Part model, mm, in its own coordinate system. Give positions to 0.01 mm unless a question says otherwise; leave off trailing zeros. Loops run counter-clockwise (first coordinate to the right, second up) from the corner with the lowest first, then second, coordinate; pieces in that order, holes last. Notation, with made-up numbers: (-27.75, -26.75) -> (2.25, -26.75) arc R24 cw to (2.25, 4.25) -> close; hole circle Ø3 at (53, -16.5). An arc over 180 degrees is marked (long way). One line per question, with ' | ' between items.
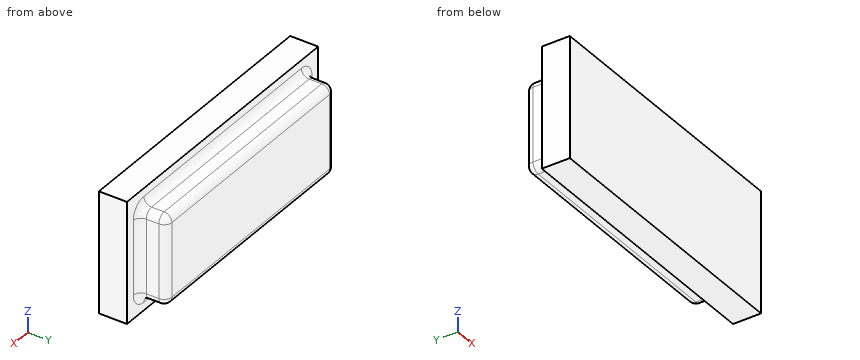
```python
from build123d import *

# Parameters (mm, degrees)
F0_W     = 199.9996
F0_H     = 86.2838
F1_DEPTH = 19.9898
F2_W     = 175.8382518563
F2_H     = 63.7771419656
F3_DEPTH = 19.9898
F4_R     = 5.5188922036


# Not quite as in the source:
# - the program builds the solid bodies; features that only make, move or delete a surface that nothing else refers to are left out


with BuildPart() as f1:
    # F0 (on Front) → F1 (new body)
    with BuildSketch(Plane.XZ):
        with Locations((27.3758191615, -15.038352045)):
            Rectangle(F0_W, F0_H)
    extrude(amount=F1_DEPTH)

    # F2 (on face) → F3 (join)
    with BuildSketch(Plane(origin=(0, 0, 0), x_dir=(-1, 0, 0), z_dir=(0, 1, 0))):
        with Locations((-27.3758191615, -15.038352045)):
            Rectangle(F2_W, F2_H)
    extrude(amount=F3_DEPTH)

    # F4
    f4_edges = [f1.edges().sort_by_distance(p)[0] for p in [
        (-60.543307, 9.9949, 16.850219),
        (115.294945, 9.9949, 16.850219),
        (27.375819, 0, 16.850219),
        (27.375819, 19.9898, 16.850219),
        (115.294945, 9.9949, -46.926923),
        (-60.543307, 9.9949, -46.926923),
        (27.375819, 0, -46.926923),
        (27.375819, 19.9898, -46.926923),
        (-60.543307, 0, -15.038352),
        (-60.543307, 19.9898, -15.038352),
        (115.294945, 0, -15.038352),
        (115.294945, 19.9898, -15.038352),
    ]]
    fillet(f4_edges, radius=F4_R)


solid = f1.part
```
1) Saw through at A-A (z = -37). Give the cut face in (x, y).
Found:
outline: (-72.62, -19.99) -> (127.38, -19.99) -> (127.38, 0) -> (120.81, 0) arc R5.52 cw to (115.29, 5.52) -> (115.29, 14.47) arc R5.52 ccw to (109.78, 19.99) -> (-55.02, 19.99) arc R5.52 ccw to (-60.54, 14.47) -> (-60.54, 5.52) arc R5.52 cw to (-66.06, 0) -> (-72.62, 0) -> close
2) Pin check, flat tips, straight feed: P1, Ø10, axis at y = 11, z = -19, coming from the +X side; P2, Ø5, axis at y = 9, z = -49, coming from the -X side; P3, Ø12, axis at x = 69, y = 10, coming from the -Z side. Stop position of each tip, or through.
Found:
P1: x = 115.29 | P2: x = -57.15 | P3: z = -47.14
3) Saw through at C-C (y = 9.5). Give the cut face in (x, z).
Found:
outline: (-60.54, -41.41) arc R5.52 ccw to (-55.02, -46.93) -> (109.78, -46.93) arc R5.52 ccw to (115.29, -41.41) -> (115.29, 11.33) arc R5.52 ccw to (109.78, 16.85) -> (-55.02, 16.85) arc R5.52 ccw to (-60.54, 11.33) -> close
4) Drill centre lines: line 1 (Z direction, x = 8.5, y = 6); line 2 (X direction, y = 8.5, z = -8); line 3 (Y direction, x = 5, z = 17.5). Where is each one in solid material? Low to high.
Found:
line 1: -46.93 to 16.85 | line 2: -60.54 to 115.29 | line 3: -19.99 to 2.92
5) Saw through at B-B (x = -31.5). Give the cut face in (y, z).
Found:
outline: (-19.99, -58.18) -> (0, -58.18) -> (0, -52.45) arc R5.52 cw to (5.52, -46.93) -> (14.47, -46.93) arc R5.52 ccw to (19.99, -41.41) -> (19.99, 11.33) arc R5.52 ccw to (14.47, 16.85) -> (5.52, 16.85) arc R5.52 cw to (0, 22.37) -> (0, 28.1) -> (-19.99, 28.1) -> close
